The model under review builds one solid part; all positions refer to its coordinate system, in mm. A direction names the side the tool comes from. Round coordinates to 2 decimals unless told otherwise and drop trailing zeros. Write each loop counter-clockwise with the first axis right and the second up, starting at its lowest first coordinate (ties: lowest second). Pieces come first, ordered by that corner, then holes. Notation, with made-up numbers: M 47,84 L 98,84 A25 cw 98,116 Z; hole C 57.5,13 d6. An arc over 180 degrees is marked long. Write item = value, one per line. Start each with the question number.
Item 1: Take a section at A-A, the plane x = 0. Give the boundary of the cut face in (y, z).
Item 2: Take a section at D-D, the plane z = 16.5. Give the boundary of the cut face in (x, y).
Item 3: The part is to be moulded in two halves that separate along X. For faces 1 (the flat face through (-8, 3, -8)), 2 (the cylindrical face through (-36.1, 1.48, -11.37)), 3 (the cylindrical face through (37.312, -7.395, -1.352)), say which applies: +X half, -X half, draft (parallel to the pull), parting line (faces both ways), or undercut.
Item 4: Take a section at B-B, the plane z = 1.5. Give the boundary of the cut face in (x, y), plus the area to 3 significant figures.
Item 5: Take a section at C-C, the plane y = -9. Give the boundary of the cut face in (x, z).
Item 6: Tool access review of faces 4 (the cylindrical face through (-28.728, -7.395, -1.352)), 5 (the flat face through (0, 2, -36)), 6 (the flat face through (31, -15, 3)): name each direction out of +Z, -Z, +X, -X, +Y, -Y from which nothing blocks a thin tool from reaching the whole face with its end or side.
Item 7: To check wall thickness, follow line 1 along Z through (x, y) = (33.02, -2); line 2 along Y through (x, z) = (-14, -23.5); line 3 along Z through (x, y) = (31.5, -2). State the ranges of each line that lie inside material, in increasing order.
Item 8: For pin 1 Ø1.5 at (x, y) = (0, 1.5) entering from -Z; pin 2 Ø2 at (x, z) = (6.5, -30) entering from -Y; pin 3 Ø3.5 at (y, z) = (1, -33.5) entering from +X, all flat-tipped, find the tip position at first contact; note any pin that passes through.
Autodesk Inventor part; units mm, degrees
ref_plane "YZ Plane" through (0, 0, 0) normal (1, 0, 0) x (0, 1, 0)
ref_plane "XZ Plane" through (0, 0, 0) normal (0, 1, 0) x (-1, 0, 0)
ref_plane "XY Plane" through (0, 0, 0) normal (0, 0, 1) x (1, 0, 0)
sketch "Sketch1" plane through (0, 0, 0) normal (0, 1, 0) x (-1, 0, 0)
  circle A0 centre (0, 0) radius 37.85
  dimension "d0" = 75.7
extrude "Extrusion1" add sketch "Sketch1" along normal blind 3
sketch "Sketch2" plane through (0, 3, 0) normal (0, 1, 0) x (1, 0, 0)
  circle A0 centre (-33.02, 0) radius 3.4
  point P0 (0, 0)
  point P1 (0, 0)
  dimension "d3" = 33.02
  dimension "d4" = 6.8
extrude "Extrusion2" cut sketch "Sketch2" against normal through all
mirror "Mirror1" about plane through (0, 0, 0) normal (1, 0, 0) of "Extrusion2"
sketch "Sketch3" plane through (0, 0, 0) normal (0, -1, 0) x (1, 0, 0)
  circle A0 centre (-33.02, 0) radius 3.4
  circle A1 centre (33.02, 0) radius 3.4
  circle A2 centre (-33.02, 0) radius 4.5
  circle A3 centre (33.02, 0) radius 4.5
  point P0 (0, 0)
  dimension "d7" = 9
  dimension "d8" = 9
extrude "Extrusion3" add sketch "Sketch3" along normal blind 15
sketch "Sketch4" plane through (0, 3, 0) normal (0, 1, 0) x (1, 0, 0)
  circle A0 centre (0, -9.736) radius 19
  point P0 (0, 0)
  dimension "d11" = 9.736
  dimension "d12" = 38
extrude "Extrusion4" cut sketch "Sketch4" against normal blind 18.5
sketch "Sketch5" plane through (0, 3, 0) normal (0, 1, 0) x (1, 0, 0)
  circle A0 centre (0, 8.554) radius 21
  point P0 (0, 0)
  dimension "d15" = 8.554
  dimension "d16" = 42
extrude "Extrusion5" [suppressed]
sketch "Sketch6" plane through (0, 3, 0) normal (0, 1, 0) x (1, 0, 0)
  line L0 (5, 36) -> (-5, 36)
  line L1 (-5, 36) -> (-5, 32.5)
  line L2 (-5, 32.5) -> (5, 32.5)
  line L3 (5, 32.5) -> (5, 36)
  circle A0 centre (0, 0) radius 37.85
  dimension "d19" = 10
  dimension "d20" = 5
  dimension "d21" = 3.5
  dimension "d22" = 36
extrude "Extrusion6" cut sketch "Sketch6" against normal through all contours L3 L2 L1 L0
equation "\"d8\" = d7"
properties part number "plate_r1"
Response values:
q1.outline = M 0,-37.85 L 3,-37.85 L 3,-36 L 0,-36 Z; M 0,-32.5 L 3,-32.5 L 3,-9.26 L 0,-9.26 Z; M 0,28.74 L 3,28.74 L 3,37.85 L 0,37.85 Z
q2.outline = M -34.06,0 L -17.76,0 L -17.76,3 L -34.06,3 Z; M 17.76,0 L 34.06,0 L 34.06,3 L 17.76,3 Z
q3.face_1 = draft
q3.face_2 = parting line
q3.face_3 = undercut
q4.outline = M -37.82,0 L -37.26,0 L -37.26,-15 L -36.07,-15 L -36.07,3 L -37.82,3 Z; M -29.97,-15 L -28.78,-15 L -28.78,0 L -17.12,0 L -17.12,3 L -29.97,3 Z; M 17.12,0 L 28.78,0 L 28.78,-15 L 29.97,-15 L 29.97,3 L 17.12,3 Z; M 36.07,-15 L 37.26,-15 L 37.26,0 L 37.82,0 L 37.82,3 L 36.07,3 Z
q4.area = 159 mm2
q5.outline = C -33.02,0 d9; C 33.02,0 d9; hole C -33.02,0 d6.8; hole C 33.02,0 d6.8
q6.face_4 = -Y
q6.face_5 = +Y, -Y
q6.face_6 = +Z, -Z, +X, -X, -Y
q7.line_1 = -4.5 to -3.4, 3.4 to 4.5
q7.line_2 = 0 to 3
q7.line_3 = -4.24 to -3.04, 3.04 to 4.24
q8.pin_1 = -37.85
q8.pin_2 = 0
q8.pin_3 = 20.6
